The listing builds one solid part. Answer for the finished solid, in the listing's coordinates (mm). A direction names the side the tool comes from. Round coordinates to 2 decimals unless told otherwise and drop trailing zeros. Order: outer loops, then holes, each group sorted by start corner. A loop starts at its lowest first (then second) coordinate and runs counter-clockwise, first axis right, second up. Notation, with made-up numbers: (-25, 68) - (17, 68) arc R12 ccw to (17, 80) - close; hole circle Ø8 at (18, 76). An arc over 180 degrees is marked (long way). One line per item, written item: value. Start each with the question number.
1. A tool of negligible diameter and unlimited length cuts with its end or side. For faces 1 (the flat face through (35, 3, -35)), 2 (the flat face through (82, 57, -66)), 3 (the flat face through (57, 65, -36)), from which of +Z, -Z, +X, -X, +Y, -Y can it reach the whole face along a straight path? Write none if from no direction.
2. Straight lines are drawn through the part: line 1 (X direction, y = 9.15, z = -23); line 2 (X direction, y = 21.5, z = -26); line 3 (Y direction, x = 99.5, z = -12). For each, find the intervals that lie inside material, in ascending order.
3. Section B-B, the plane x = 20 is taken. Give the vertices of the cut face in (y, z).
4. For a pull along X with two mould halves and no side action, classify faces 4 (the flat face through (148, 12, -36)), 5 (the cylindrical face through (67.79, 77.32, -55.34)), 6 (the flat face through (35, 34, -36)), 7 (the cylindrical face through (119.29, 50.33, -35.07)) as released by +X, released by -X, zero draft, split by the parting line, or undercut.
5. Section D-D, the plane z = -63.5 is taken. Give the vertices of the cut face in (x, y), then the cut area to 3 significant figures.
6. Flat-ended cylindrical pins translate along their axes: P1, Ø20, axis at x = 142, z = -21.5, coming from the -Y side; P2, Ø4, axis at x = 37.5, z = -46.5, coming from the +Y side; P3, Ø19, axis at x = 20, z = -23, coming from the +Y side; P4, Ø11, axis at x = 20, z = -48, coming from the +Y side. Find the tip coordinate at first contact, or state that the pin passes through.
7. Section C-C, the plane x = 83 is taken. Give the vertices of the cut face in (y, z).
from build123d import *

# Parameters (mm, degrees)
SKETCH1_W           = 166
SKETCH1_H           = 71
BOSS_EXTRUDE1_DEPTH = 12
SKETCH2_R           = 6
CUT_EXTRUDE1_DEPTH  = 181.944742947
SKETCH3_W           = 96
SKETCH3_H           = 71
BOSS_EXTRUDE2_DEPTH = 53
SKETCH4_W           = 25
SKETCH4_H           = 6
CUT_EXTRUDE2_DEPTH  = 192.890593829
SKETCH5_W           = 5
SKETCH5_H           = 53
CUT_EXTRUDE4_DEPTH  = 163.563833616
BOSS_EXTRUDE4_DEPTH = 10
BOSS_EXTRUDE5_START = -10
BOSS_EXTRUDE5_DEPTH = 10
FILLET4_R           = 10
FILLET5_R           = 10
SKETCH11_R          = 25
SKETCH11_R_2        = 12.5
BOSS_EXTRUDE6_DEPTH = 25
SKETCH12_R          = 12.5
CUT_EXTRUDE5_DEPTH  = 192.890593829


with BuildPart() as part:
    # Sketch1 → Boss-Extrude1 (new body)
    with BuildSketch(Plane(origin=(0, 0, 0), x_dir=(1, 0, 0), z_dir=(0, 1, 0))):
        with Locations((83, 35.5)):
            Rectangle(SKETCH1_W, SKETCH1_H)
    extrude(amount=BOSS_EXTRUDE1_DEPTH)

    # Sketch2 → Cut-Extrude1 (cut, through all)
    with BuildSketch(Plane(origin=(0, 12, 0), x_dir=(1, 0, 0), z_dir=(0, 1, 0))):
        with Locations(Location((20, 48, 0), (0, 0, 270))):
            Circle(SKETCH2_R)
        with Locations(Location((20, 23, 0), (0, 0, 270))):
            Circle(SKETCH2_R)
        with Locations(Location((146, 48, 0), (0, 0, 270))):
            Circle(SKETCH2_R)
        with Locations(Location((146, 23, 0), (0, 0, 270))):
            Circle(SKETCH2_R)
    extrude(amount=-CUT_EXTRUDE1_DEPTH, mode=Mode.SUBTRACT)

    # Sketch3 → Boss-Extrude2 (add)
    with BuildSketch(Plane(origin=(0, 12, 0), x_dir=(1, 0, 0), z_dir=(0, 1, 0))):
        with Locations((83, 35.5)):
            Rectangle(SKETCH3_W, SKETCH3_H)
    extrude(amount=BOSS_EXTRUDE2_DEPTH)

    # Sketch4 → Cut-Extrude2 (cut, through all)
    with BuildSketch(Plane.XY):
        with BuildLine():
            Line((45, 0), (121, 0))
            Line((121, 0), (121, 46.135540556))
            ThreePointArc((121, 46.135540556), (119.242640687, 50.378181243), (115, 52.135540556))
            Line((115, 52.135540556), (51, 52.135540556))
            ThreePointArc((51, 52.135540556), (46.757359313, 50.378181243), (45, 46.135540556))
            Line((45, 46.135540556), (45, 0))
        make_face()
        with Locations((22.5, 3)):
            Rectangle(SKETCH4_W, SKETCH4_H)
        with Locations((143.5, 3)):
            Rectangle(SKETCH4_W, SKETCH4_H)
    extrude(amount=-CUT_EXTRUDE2_DEPTH, mode=Mode.SUBTRACT)

    # Sketch5 → Cut-Extrude4 (cut, through all)
    with BuildSketch(Plane.ZY.offset(-35)):
        with Locations((-68.5, 38.5)):
            Rectangle(SKETCH5_W, SKETCH5_H)
        with Locations((-2.5, 38.5)):
            Rectangle(SKETCH5_W, SKETCH5_H)
    extrude(amount=-CUT_EXTRUDE4_DEPTH, mode=Mode.SUBTRACT)

    # Sketch7 → Boss-Extrude4 (add)
    with BuildSketch(Plane.ZY.offset(-35)):
        with BuildLine():
            Line((-71, 12), (-66, 12))
            Line((-66, 12), (-66, 19.610148588))
            ThreePointArc((-66, 19.610148588), (-67.361838539, 15.057282415), (-71, 12))
        make_face()
        with BuildLine():
            Line((-5, 20.660254038), (-5, 12))
            Line((-5, 12), (0, 12))
            ThreePointArc((0, 12), (-3.660254038, 15.660254038), (-5, 20.660254038))
        make_face()
    extrude(amount=-BOSS_EXTRUDE4_DEPTH)

    # Sketch10 → Boss-Extrude5 (add)
    with BuildSketch(Plane(origin=(131, 0, 0), x_dir=(0, 0, -1), z_dir=(1, 0, 0)).offset(BOSS_EXTRUDE5_START)):
        with BuildLine():
            Line((5, 20.660254038), (5, 12))
            Line((5, 12), (0, 12))
            ThreePointArc((0, 12), (3.660254038, 15.660254038), (5, 20.660254038))
        make_face()
        with BuildLine():
            Line((71, 12), (66, 12))
            Line((66, 12), (66, 19.610148588))
            ThreePointArc((66, 19.610148588), (67.361838539, 15.057282415), (71, 12))
        make_face()
    extrude(amount=BOSS_EXTRUDE5_DEPTH)

    # Fillet4
    fillet4_edges = [part.edges().sort_by_distance(p)[0] for p in [
        (35, 65, -35.5),
    ]]
    fillet(fillet4_edges, radius=FILLET4_R)

    # Fillet5
    fillet5_edges = [part.edges().sort_by_distance(p)[0] for p in [
        (131, 65, -35.5),
    ]]
    fillet(fillet5_edges, radius=FILLET5_R)

    # Sketch11 → Boss-Extrude6 (add)
    with BuildSketch(Plane(origin=(0, 65, 0), x_dir=(1, 0, 0), z_dir=(0, 1, 0))):
        with Locations(Location((83, 35.5, 0), (0, 0, 270))):
            Circle(SKETCH11_R)
        with Locations(Location((83, 35.5, 0), (0, 0, 270))):
            Circle(SKETCH11_R_2, mode=Mode.SUBTRACT)
    extrude(amount=BOSS_EXTRUDE6_DEPTH)

    # Sketch12 → Cut-Extrude5 (cut, through all)
    with BuildSketch(Plane(origin=(0, 65, 0), x_dir=(1, 0, 0), z_dir=(0, 1, 0))):
        with Locations(Location((83, 35.5, 0), (0, 0, 270))):
            Circle(SKETCH12_R)
    extrude(amount=-CUT_EXTRUDE5_DEPTH, mode=Mode.SUBTRACT)


solid = part.part
Answer list:
1. face 1: +Z, -Z, -Y
1. face 2: -Z, +X, -X, +Y
1. face 3: +Y
2. line 1: x = 0 to 14, 26 to 45, 121 to 140, 152 to 166
2. line 2: x = 35 to 45, 121 to 131
2. line 3: y = 52.14 to 65
3. outline: (6, -71) - (12, -71) - (12, -54) - (6, -54) - close; (6, -42) - (12, -42) - (12, -29) - (6, -29) - close; (6, -17) - (12, -17) - (12, 0) - (6, 0) - close
4. face 4: zero draft
4. face 5: split by the parting line
4. face 6: released by -X
4. face 7: undercut
5. outline: (0, 0) - (10, 0) - (10, 6) - (35, 6) - (35, 0) - (45, 0) - (45, 46.14) arc R6 cw to (51, 52.14) - (115, 52.14) arc R6 cw to (121, 46.14) - (121, 0) - (131, 0) - (131, 6) - (156, 6) - (156, 0) - (166, 0) - (166, 12) - (131, 12) - (131, 55) arc R10 ccw to (121, 65) - (45, 65) arc R10 ccw to (35, 55) - (35, 12) - (0, 12) - close
5. area: 2,790 mm²
6. P1: stops at y = 6
6. P2: stops at y = 63.35
6. P3: stops at y = 12
6. P4: passes through
7. outline: (52.14, -66) - (65, -66) - (65, -60.5) - (90, -60.5) - (90, -48) - (52.14, -48) - close; (52.14, -23) - (90, -23) - (90, -10.5) - (65, -10.5) - (65, -5) - (52.14, -5) - close
